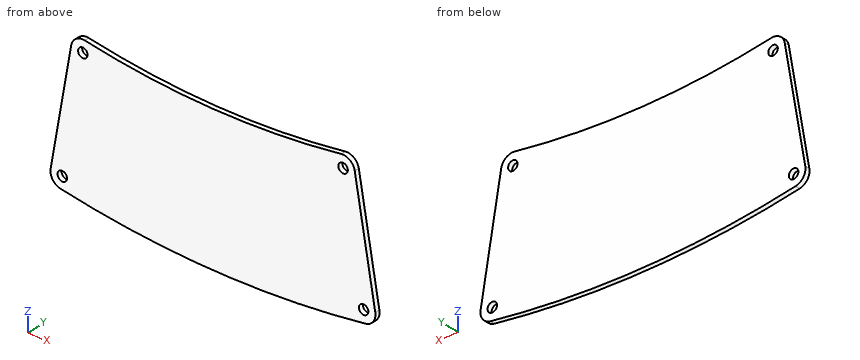
from build123d import *

# Parameters (mm, degrees)
SM_BASE_FLANGE_1_DEPTH = 2
FILLET_1_R             = 5
SKETCH_2_R             = 2
CUT_EXTRUDE_1_DEPTH    = 10


# Sheet-metal steps are written as plain solids
with BuildPart() as part:
    # Sketch 1 → Базовая кромка1 (new body)
    with BuildSketch(Plane(origin=(0, 0, 0), x_dir=(1, 0, 0), z_dir=(0, 1, 0))):
        with BuildLine():
            Line((-59.040380407, 334.834636024), (-69.459271067, 393.923101205))
            ThreePointArc((-69.459271067, 393.923101205), (0, 400), (69.459271067, 393.923101205))
            Line((69.459271067, 393.923101205), (59.040380407, 334.834636024))
            ThreePointArc((59.040380407, 334.834636024), (0, 340), (-59.040380407, 334.834636024))
        make_face()
    extrude(amount=-SM_BASE_FLANGE_1_DEPTH)

    # Скругление1
    fillet_1_edges = [part.edges().sort_by_distance(p)[0] for p in [
        (-59.040380407, -1, -334.834636024),
        (-69.459271067, -1, -393.923101205),
        (69.459271067, -1, -393.923101205),
        (59.040380407, -1, -334.834636024),
    ]]
    fillet(fillet_1_edges, radius=FILLET_1_R)

    # Эскиз2 → Вырез-Вытянуть1 (cut)
    with BuildSketch(Plane(origin=(0, 0, 0), x_dir=(1, 0, 0), z_dir=(0, 1, 0))):
        with Locations(Location((-63.661495998, 389.836137277, 0), (0, 0, 270))):
            Circle(SKETCH_2_R)
        with Locations(Location((-54.978290599, 340.591232363, 0), (0, 0, 270))):
            Circle(SKETCH_2_R)
        with Locations(Location((63.661495998, 389.836137277, 0), (0, 0, 270))):
            Circle(SKETCH_2_R)
        with Locations(Location((54.978290599, 340.591232363, 0), (0, 0, 270))):
            Circle(SKETCH_2_R)
    extrude(amount=-CUT_EXTRUDE_1_DEPTH, mode=Mode.SUBTRACT)


solid = part.part
Work out the finished part from the listing and answer in its coordinate system (mm). Coordinates: 2 decimals unless noted, no trailing zeros. Write each loop counter-clockwise with the first axis right and the second up, starting at its lowest first coordinate (ties: lowest second). Pieces come first, ordered by that corner, then holes.
1. The part is cut by section A-A, the plane y = -1.55. Write down the section's boundary in (x, z), and give its area (3 significant figures).
Results list:
outline: (-68.59, -388.97) arc R5 ccw to (-64.47, -394.77) arc R400 ccw to (64.47, -394.77) arc R5 ccw to (68.59, -388.97) - (59.9, -339.72) arc R5 ccw to (54.18, -335.66) arc R340 cw to (-54.18, -335.66) arc R5 ccw to (-59.9, -339.72) - close; hole circle Ø4 at (-63.66, -389.84); hole circle Ø4 at (-54.98, -340.59); hole circle Ø4 at (54.98, -340.59); hole circle Ø4 at (63.66, -389.84)
area: 7,680 mm2
2. The part is cut by section C-C, the plane x = 28. Write down the section's boundary in (y, z).
Results list:
outline: (-2, -399.02) - (0, -399.02) - (0, -338.85) - (-2, -338.85) - close
3. A flat-ended cylindrical pin translates along its axis: pin 1 (4.5 mm diameter, centred on x = 54.98, z = -340.59, fed in from +Y). Find the tip coordinate at first contact, or state that the pin passes through.
Results list:
pin 1: stops at y = 0
4. Consider line 1 along Z through (x, y) = (-8.5, -0.4); line 2 along X through (y, z) = (-0.5, -347.5); line 3 along Z through (x, y) = (-26, -1.7). Determine where each line is inside the solid, lowest interval first.
Results list:
line 1: z = -399.91 to -339.89
line 2: x = -61.27 to 61.27
line 3: z = -399.15 to -339
5. The part is cut by section B-B, the plane z = -379. Write down the section's boundary in (x, y), and give its area (3 significant figures).
Results list:
outline: (-66.83, -2) - (66.83, -2) - (66.83, 0) - (-66.83, 0) - close
area: 267 mm2
